```python
from build123d import *

# Parameters (mm, degrees)
SKETCH1_W           = 17
SKETCH1_H           = 60
BOSS_EXTRUDE1_DEPTH = 5
SKETCH2_W           = 17
SKETCH2_H           = 5
BOSS_EXTRUDE2_DEPTH = 7
SKETCH3_W           = 17
SKETCH3_H           = 5
BOSS_EXTRUDE3_DEPTH = 75
SKETCH4_R           = 1.6
CUT_EXTRUDE1_DEPTH  = 106.575802152
CUT_EXTRUDE2_DEPTH  = 2


with BuildPart() as part:
    # Sketch1 → Boss-Extrude1 (new body)
    with BuildSketch(Plane.XY):
        Rectangle(SKETCH1_W, SKETCH1_H)
        with BuildLine():
            Line((0.1, 20), (0.1, -25))
            ThreePointArc((0.1, -25), (-1.5, -26.6), (-3.1, -25))
            Line((-3.1, -25), (-3.1, 20))
            ThreePointArc((-3.1, 20), (-1.5, 21.6), (0.1, 20))
        make_face(mode=Mode.SUBTRACT)
    extrude(amount=BOSS_EXTRUDE1_DEPTH)

    # Sketch2 → Boss-Extrude2 (add)
    with BuildSketch(Plane.XY.offset(5)):
        with Locations((0, 27.5)):
            Rectangle(SKETCH2_W, SKETCH2_H)
    extrude(amount=BOSS_EXTRUDE2_DEPTH)

    # Sketch3 → Boss-Extrude3 (add)
    with BuildSketch(Plane(origin=(0, 30, 0), x_dir=(1, 0, 0), z_dir=(0, 1, 0))):
        with Locations((0, -9.5)):
            Rectangle(SKETCH3_W, SKETCH3_H)
    extrude(amount=BOSS_EXTRUDE3_DEPTH)

    # Sketch4 → Cut-Extrude1 (cut, through all)
    with BuildSketch(Plane(origin=(0, 0, 7), x_dir=(-1, 0, 0), z_dir=(0, 0, -1))):
        with Locations((0, 96.5)):
            Circle(SKETCH4_R)
    extrude(amount=-CUT_EXTRUDE1_DEPTH, mode=Mode.SUBTRACT)

    # Sketch5 → Cut-Extrude2 (cut)
    with BuildSketch(Plane(origin=(0, 0, 0), x_dir=(-1, 0, 0), z_dir=(0, 0, -1))):
        Polygon((-0.5, 21.6), (-0.5, 30), (-8.5, 30), (-8.5, 16), (-0.5, 16), align=None)
        with BuildLine():
            Line((1.5, 21.6), (-0.5, 21.6))
            Line((-0.5, 21.6), (-0.5, 16))
            Line((-0.5, 16), (-0.1, 16))
            Line((-0.1, 16), (-0.1, 20))
            ThreePointArc((-0.1, 20), (0.36862915, 21.13137085), (1.5, 21.6))
        make_face()
        Polygon((-0.5, -21), (-8.5, -21), (-8.5, -30), (-0.5, -30), (-0.5, -26.6), align=None)
        with BuildLine():
            Line((-0.1, -21), (-0.5, -21))
            Line((-0.5, -21), (-0.5, -26.6))
            Line((-0.5, -26.6), (1.5, -26.6))
            ThreePointArc((1.5, -26.6), (0.36862915, -26.13137085), (-0.1, -25))
            Line((-0.1, -25), (-0.1, -21))
        make_face()
    extrude(amount=-CUT_EXTRUDE2_DEPTH, mode=Mode.SUBTRACT)


solid = part.part
```
Geometry: final body of the model. Coordinates: model frame, mm. A direction names the side the tool comes from. Coordinates: 2 decimals unless noted, no trailing zeros. Order: outer loops, then holes, each group sorted by start corner. A loop starts at its lowest first (then second) coordinate and runs counter-clockwise, first axis right, second up. Notation, with made-up numbers: M 4.5,82 L 61.5,82 A23 cw 61.5,91 Z; hole C -19.5,-17 d5. An arc over 180 degrees is marked long. Answer as CSV lines item,"result".
Q1. Line query: probe 1 along Y at (x, z) = (0, 9.15); probe 2 along X at (y, z) = (-0.5, 2.5); probe 3 along X at (y, z) = (96.5, 10.25). Output: solid intervals per line, ascending. Write a range as [from, to].
Answers:
probe 1,"y = [25, 94.9], [98.1, 105]"
probe 2,"x = [-8.5, -3.1], [0.1, 8.5]"
probe 3,"x = [-8.5, -1.6], [1.6, 8.5]"
Q2. Section B-B on z = 3.75. Return the cut outline in (x, y), and give its area (3 significant figures).
Answers:
outline,"M -8.5,-30 L 8.5,-30 L 8.5,30 L -8.5,30 Z; hole M -3.1,-25 A1.6 ccw 0.1,-25 L 0.1,20 A1.6 ccw -3.1,20 Z"
area,"868 mm^2"
Q3. Draft query along X for faces 4 (the cylindrical face through (-2.08, 21.49, 3.02)), 5 (the cylindrical face through (-2.014, -26.515, 3.021)), 6 (the flat face through (5, 23, 2)), 7 (the flat face through (-8.5, 36.6, 7.4)). Return one class per face: pulls with the +X half, pulls with the -X half, needs draft (parallel to the pull), parting line crosses it, or undercut.
Answers:
face 4,"undercut"
face 5,"undercut"
face 6,"needs draft"
face 7,"pulls with the -X half"
Q4. Section C-C on x = -4.75. Return the cut outline in (y, z).
Answers:
outline,"M -30,0 L 30,0 L 30,7 L 105,7 L 105,12 L 25,12 L 25,5 L -30,5 Z"
Q5. Section D-D on y = 27.5. Return the cut outline in (x, z).
Answers:
outline,"M -8.5,0 L 0.5,0 L 0.5,2 L 8.5,2 L 8.5,12 L -8.5,12 Z"
Q6. Section A-A on y = 96.5. Return the cut outline in (x, z), and give its area (3 significant figures).
Answers:
outline,"M -8.5,7 L -1.6,7 L -1.6,12 L -8.5,12 Z; M 1.6,7 L 8.5,7 L 8.5,12 L 1.6,12 Z"
area,"69.0 mm^2"
Q7. Set-up query: faces 1 (the flat face through (0, 67, 7)), 2 (the flat face through (0, 25, 8)), 3 (the flat face through (-3.1, -3, 2)). Return all of +Z, -Z, +X, -X, +Y, -Y with unobstructed straight access to the full face (end or side cutting, diameter ignored); none if empty.
Answers:
face 1,"-Z, +X, -X, +Y"
face 2,"+Z, +X, -X, -Y"
face 3,"+Z, -Z"
Q8. First-contact query: P1, Ø5, axis at x = 5, y = -10.5, coming from the +Z side; P2, Ø5, axis at x = 0, y = 96.5, coming from the -Z side; P3, Ø3.5, axis at x = -3, z = 4.5, coming from the +Y side; P4, Ø8, axis at x = -5, y = 30.5, coming from the -Z side. Flat tips, straight axial feed; report the tip coordinate or a pass-through.
Answers:
P1,"stops at z = 5"
P2,"stops at z = 7"
P3,"stops at y = 30"
P4,"stops at z = 0"
